Check sheet for the drawn part. Datum: minimum x, y, z corner. Units: mm. A direction names the side the tool comes from. Round coordinates to 2 decimals unless told otherwise and drop trailing zeros. Write each loop counter-clockwise with the first axis right and the second up, starting at its lowest first coordinate (ties: lowest second). Pieces come first, ordered by that corner, then holes. Notation, with made-up numbers: M -10,26.25 L 21,26.25 A25 cw 21,61.25 Z; hole C -30.5,24.25 d6. An arc over 180 degrees is marked long. One line per item, written item: value. Start each with the question number.
Item 1: Section check C-C, the plane z = 17.5. Record the cut outline in (x, y).
Item 2: Tool access check on the marked faces 4 and 5. Record the directions out of +Z, -Z, +X, -X, +Y, -Y that give a thin tool (end or side, any length) a straight path to the whole face; none if there is none.
Item 3: Gauge pin test, flat ends, axial feed: pin 1 (10 mm diameter, centred on y = 29.5, z = 28.5, fed in from +X); pin 2 (6 mm diameter, centred on x = 28, y = 37.5, fed in from +Z); pin 3 (2 mm diameter, centred on x = 30, z = 30, fed in from -Y); pin 4 (5 mm diameter, centred on x = 24, z = 29, fed in from +Y). Record the tip position at first contact, or that the pin passes through.
Item 4: Thickness scan on probe 1 along Z at (x, y) = (5, 2.5); probe 2 along X at (y, z) = (4, 30); probe 3 along Y at (x, z) = (28, 20.5). Record the ranges inside material, lowest first. Write a range as from..to.
Item 5: Draft check along Z on the marked faces 1, 2 and 3. Enter one of: +Z half, -Z half, draft (parallel to the pull), parting line (faces both ways), or undercut.
Item 6: Section check A-A, the plane y = 4.5. Record the cut outline in (x, z).
Item 7: Section check B-B, the plane x = 17.5. Record the cut outline in (y, z).
Item 8: Section check D-D, the plane y = 15.5. Record the cut outline in (x, z), then the cut area to 3 significant figures.
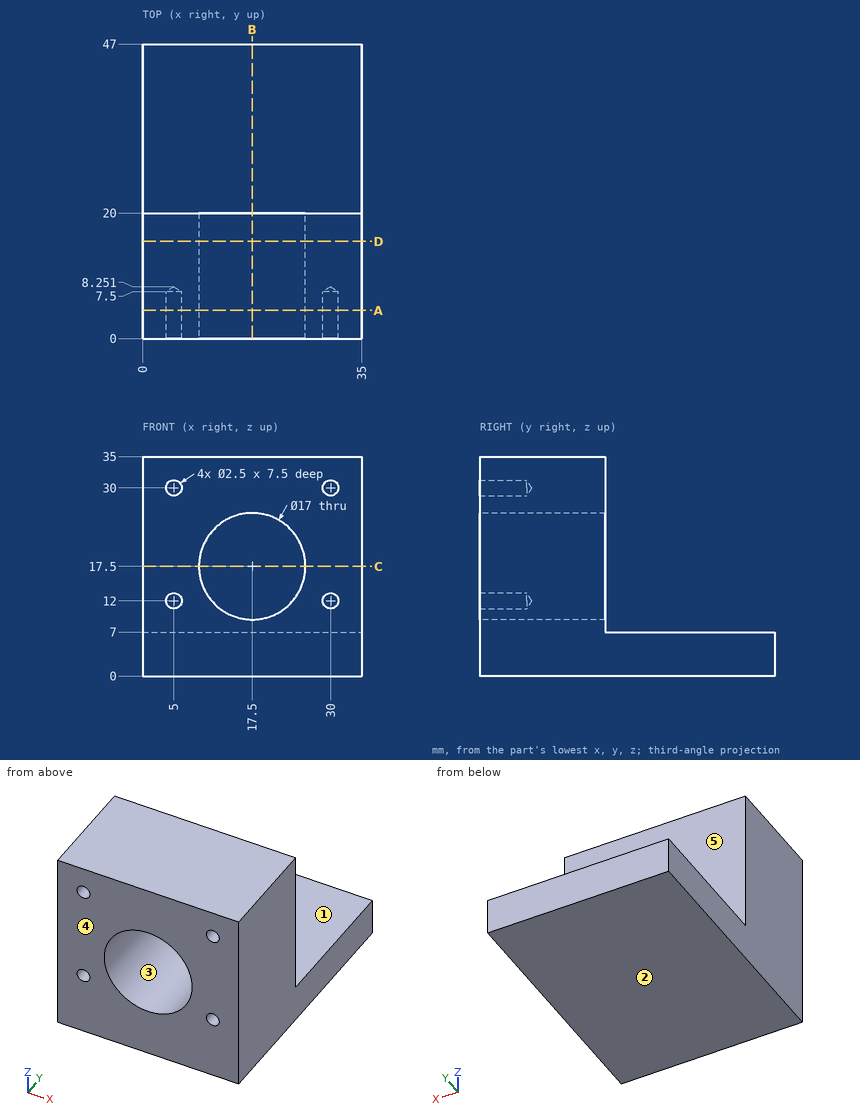
Response values:
1. outline: M 0,0 L 9,0 L 9,20 L 0,20 Z; M 26,0 L 35,0 L 35,20 L 26,20 Z
2. face 4: +Z, -Z, +X, -X, -Y
2. face 5: +Z, +X, -X, +Y
3. pin 1: passes through
3. pin 2: stops at z = 7
3. pin 3: stops at y = 7.65
3. pin 4: stops at y = 20
4. probe 1: z = 0..10.75, 13.25..28.75, 31.25..35
4. probe 2: x = 0..3.75, 6.25..28.75, 31.25..35
4. probe 3: y = 0..20
5. face 1: +Z half
5. face 2: -Z half
5. face 3: undercut
6. outline: M 0,0 L 35,0 L 35,35 L 0,35 Z; hole C 5,12 d2.5; hole C 5,30 d2.5; hole C 17.5,17.5 d17; hole C 30,12 d2.5; hole C 30,30 d2.5
7. outline: M 0,0 L 47,0 L 47,7 L 20,7 L 20,9 L 0,9 Z; M 0,26 L 20,26 L 20,35 L 0,35 Z
8. outline: M 0,0 L 35,0 L 35,35 L 0,35 Z; hole C 17.5,17.5 d17
8. area: 998 mm2
